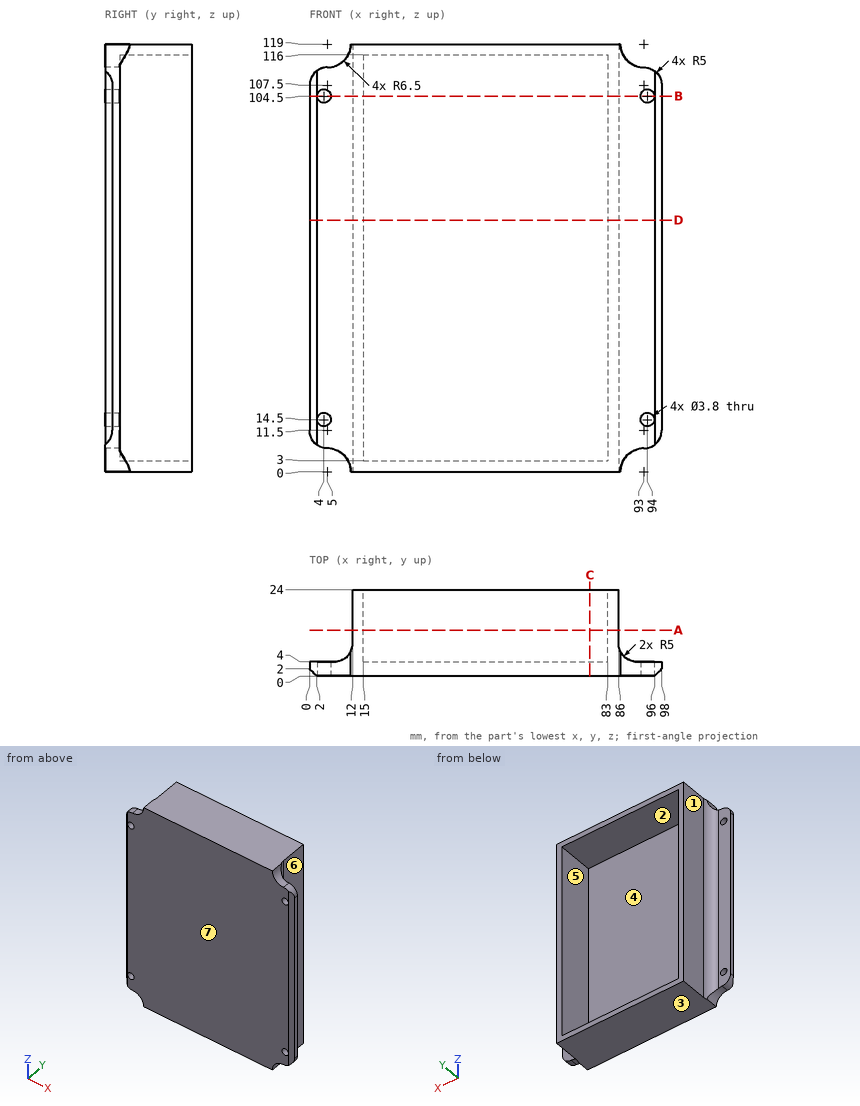
Drawing for the job (mm, zero at the part's lowest x, y, z). A direction names the side the tool comes from. Round coordinates to 2 decimals unless told otherwise and drop trailing zeros. Loops run counter-clockwise (first coordinate to the right, second up) from the corner with the lowest first, then second, coordinate; pieces in that order, holes last. Notation, with made-up numbers: (69.25, -40) - (106.25, -40) arc R13 cw to (106.25, -25) - close; hole circle Ø6 at (-9, 87.5). An arc over 180 degrees is marked (long way). Return JSON: item names as keys, results as strings. Group by question number.
Q1. Band-saw the part on C-C on x = 78. Give the cut face in (y, z).
Q2. Flat gauge pins, fed straight in: pin 1 Ø6 at (x, z) = (4, 104.5) entering from +Y; pin 2 Ø10 at (y, z) = (16, 51.5) entering from -X; pin 3 Ø7.5 at (x, z) = (4.5, 55.5) entering from +Y; pin 4 Ø2.5 at (x, z) = (94, 14.5) entering from +Y. Where does each tip first touch, or does it go through?
Q3. Band-saw the part on B-B on z = 104.5. Give the cut face in (x, y), plus the area to 3 significant figures.
Q4. Band-saw the part on A-A on y = 12.75. Give the cut face in (x, z).
Q5. Band-saw the part on D-D on z = 70. Give the cut face in (x, y), plus the area to 3 significant figures.
Q6. Drill centre lines: line 1 along X through (y, z) = (2.7, 104.5); line 2 along X through (y, z) = (11.75, 18.5); line 3 along Z through (x, y) = (54, 22.75). Where is each one in solid material? Low to high. Write a range as [from, to].
Q7. Tool access for the marked faces 5, 6 and 7: list every direction of +Z, -Z, +X, -X, +Y, -Y with a clear straight run to the whole face (end or side of a thin tool).
Q8. Two-plate mould, pull along Z, no slides. Class the marked faces 1, 2, 3 and 4: +Z half, -Z half, draft (parallel to the pull), parting line (faces both ways), or undercut.
Solutions:
{
 "1": {"outline": "(0, 0) - (24, 0) - (24, 3) - (4, 3) - (4, 116) - (24, 116) - (24, 119) - (0, 119) - close"},
 "2": {"pin 1": "stops at y = 4", "pin 2": "stops at x = 12", "pin 3": "stops at y = 4.16", "pin 4": "passes through"},
 "3": {"outline": "(0, 2) - (2, 0) - (2.1, 0) - (2.1, 4) - (0, 4) - close; (5.9, 0) - (92.1, 0) - (92.1, 4) - (91, 4) arc R5 cw to (86, 9) - (86, 24) - (83, 24) - (83, 4) - (15, 4) - (15, 24) - (12, 24) - (12, 9) arc R5 cw to (7, 4) - (5.9, 4) - close; (95.9, 0) - (96, 0) - (98, 2) - (98, 4) - (95.9, 4) - close", "area": "488 mm^2"},
 "4": {"outline": "(12, 0) - (86, 0) - (86, 119) - (12, 119) - close; hole (15, 3) - (83, 3) - (83, 116) - (15, 116) - close"},
 "5": {"outline": "(0, 2) - (2, 0) - (96, 0) - (98, 2) - (98, 4) - (91, 4) arc R5 cw to (86, 9) - (86, 24) - (83, 24) - (83, 4) - (15, 4) - (15, 24) - (12, 24) - (12, 9) arc R5 cw to (7, 4) - (0, 4) - close", "area": "519 mm^2"},
 "6": {"line 1": "x = [0, 2.1], [5.9, 92.1], [95.9, 98]", "line 2": "x = [12, 15], [83, 86]", "line 3": "z = [0, 3], [116, 119]"},
 "7": {"face 5": "+Y", "face 6": "+Z, -Z, +X, +Y", "face 7": "+Z, -Z, +X, -X, -Y"},
 "8": {"face 1": "draft", "face 2": "undercut", "face 3": "-Z half", "face 4": "undercut"}
}
